```python
from build123d import *

# Parameters (mm, degrees)
SKETCH_1_R          = 2.25
EXTRUDE_2_DEPTH     = 20
SKETCH_7_W          = 2.4
SKETCH_7_H          = 2.4
CUT_EXTRUDE_3_DEPTH = 2.5
SKETCH_9_R          = 3
EXTRUDE_4_DEPTH     = 1
SKETCH_10_W         = 4
SKETCH_10_H         = 4
EXTRUDE_5_DEPTH     = 2


with BuildPart() as part:
    # 草图1 → 凸台-拉伸2 (new body)
    with BuildSketch(Plane.XY):
        Circle(SKETCH_1_R)
    extrude(amount=EXTRUDE_2_DEPTH)

    # 草图7 → 切除-拉伸3 (cut)
    with BuildSketch(Plane.XY):
        Rectangle(SKETCH_7_W, SKETCH_7_H)
    extrude(amount=CUT_EXTRUDE_3_DEPTH, mode=Mode.SUBTRACT)

    # 草图9 → 凸台-拉伸4 (add)
    with BuildSketch(Plane.XY.offset(20)):
        Circle(SKETCH_9_R)
    extrude(amount=EXTRUDE_4_DEPTH)

    # 草图10 → 凸台-拉伸5 (add)
    with BuildSketch(Plane.XY.offset(21)):
        Rectangle(SKETCH_10_W, SKETCH_10_H)
    extrude(amount=EXTRUDE_5_DEPTH)


solid = part.part
```
Design review of the part built by this model. Coordinates are the model's own, in mm. A direction names the side the tool comes from. Round coordinates to 2 decimals unless told otherwise and drop trailing zeros. Write each loop counter-clockwise with the first axis right and the second up, starting at its lowest first coordinate (ties: lowest second). Pieces come first, ordered by that corner, then holes. Notation, with made-up numbers: (29.25, -3.5) -> (82.25, -3.5) arc R33 ccw to (82.25, 31.5) -> close; hole circle Ø11 at (28.5, 79). An arc over 180 degrees is marked (long way). Write item = value, one per line. Start each with the question number.
1) Take a section at A-A, the plane x = 0. State the section outline as (y, z) points.
2) Mouldability with a two-part tool opening along X and no side actions: class faces 1 (the face through (0, 2, 22)), 2 (the face through (1.2, 0, 1)), 3 (the face through (-2, 0, 22)) as +X half, -X half, draft (parallel to the pull), parting line (faces both ways), or undercut.
3) Take a section at C-C, the plane z = 9.5. State the section outline as (x, y) points, plus the area to 3 significant figures.
4) Wall thickness on probe 1 along Z at (x, y) = (-2.45, -0.5); probe 2 along Z at (x, y) = (-0.35, -0.05); probe 3 along Y at (x, z) = (0.15, 6.75) (3 decimals): over which ranges is each line inside the solid? List them lowest first. Write a range as from..to.
5) Clearance check with flat-ended pins moving along their axes: pin 1 (2.5 mm diameter, centred on x = 0.5, z = 2, fed in from +Y); pin 2 (1.2 mm diameter, centred on x = 0, z = 0.5, fed in from -Y); pin 3 (1 mm diameter, centred on y = 1, z = 22, fed in from +X). State where each tip first meets the part, or that it passes through.
6) Take a section at D-D, the plane y = -1.6. State the section outline as (x, z) points, plus the area to 3 significant figures.
7) Tool access review of faces 4 (the face through (0, -2, 22)), 5 (the face through (2, 0, 22)), 6 (the face through (0, 1.2, 1)): name each direction out of +Z, -Z, +X, -X, +Y, -Y from which nothing blocks a thin tool from reaching the whole face with its end or side.
Results list:
q1.outline = (-3, 20) -> (-2.25, 20) -> (-2.25, 0) -> (-1.2, 0) -> (-1.2, 2.5) -> (1.2, 2.5) -> (1.2, 0) -> (2.25, 0) -> (2.25, 20) -> (3, 20) -> (3, 21) -> (2, 21) -> (2, 23) -> (-2, 23) -> (-2, 21) -> (-3, 21) -> close
q2.face_1 = draft
q2.face_2 = undercut
q2.face_3 = -X half
q3.outline = circle Ø4.5 at (0, 0)
q3.area = 15.9 mm²
q4.probe_1 = 20..21
q4.probe_2 = 2.5..23
q4.probe_3 = -2.245..2.245
q5.pin_1 = 2.25
q5.pin_2 = -2.25
q5.pin_3 = 2
q6.outline = (-2.54, 20) -> (-1.58, 20) -> (-1.58, 0) -> (1.58, 0) -> (1.58, 20) -> (2.54, 20) -> (2.54, 21) -> (2, 21) -> (2, 23) -> (-2, 23) -> (-2, 21) -> (-2.54, 21) -> close
q6.area = 76.4 mm²
q7.face_4 = +Z, +X, -X, -Y
q7.face_5 = +Z, +X, +Y, -Y
q7.face_6 = -Z
